from build123d import *

# Parameters (mm, degrees)
SKETCH1_W           = 150
SKETCH1_H           = 220
SKETCH1_R           = 2
SKETCH1_R_2         = 4
SKETCH1_W_2         = 25
SKETCH1_H_2         = 120
BOSS_EXTRUDE1_DEPTH = 12
SKETCH2_R           = 2
CUT_EXTRUDE1_DEPTH  = 12


with BuildPart() as part:
    # Sketch1 → Boss-Extrude1 (new body)
    with BuildSketch(Plane(origin=(0, 0, 0), x_dir=(1, 0, 0), z_dir=(0, 1, 0))):
        Rectangle(SKETCH1_W, SKETCH1_H)
        with Locations(Location((-40, 34.75, 0), (0, 0, 270))):
            Circle(SKETCH1_R, mode=Mode.SUBTRACT)
        with Locations(Location((-40, -34.75, 0), (0, 0, 270))):
            Circle(SKETCH1_R, mode=Mode.SUBTRACT)
        with Locations(Location((-50, 90, 0), (0, 0, 270))):
            Circle(SKETCH1_R_2, mode=Mode.SUBTRACT)
        with Locations(Location((50, 90, 0), (0, 0, 270))):
            Circle(SKETCH1_R_2, mode=Mode.SUBTRACT)
        with Locations(Location((-50, -90, 0), (0, 0, 270))):
            Circle(SKETCH1_R_2, mode=Mode.SUBTRACT)
        with Locations(Location((50, -90, 0), (0, 0, 270))):
            Circle(SKETCH1_R_2, mode=Mode.SUBTRACT)
        with Locations((8, 0)):
            Rectangle(SKETCH1_W_2, SKETCH1_H_2, mode=Mode.SUBTRACT)
    extrude(amount=BOSS_EXTRUDE1_DEPTH)

    # Sketch2 → Cut-Extrude1 (cut)
    with BuildSketch(Plane(origin=(0, 12, 0), x_dir=(1, 0, 0), z_dir=(0, 1, 0))):
        with Locations(Location((32.75, 26.5, 0), (0, 0, 270))):
            Circle(SKETCH2_R)
        with Locations(Location((32.75, -5.5, 0), (0, 0, 270))):
            Circle(SKETCH2_R)
    extrude(amount=-CUT_EXTRUDE1_DEPTH, mode=Mode.SUBTRACT)


solid = part.part
For this review, take the finished solid that the model builds, in its own axes (mm). A direction names the side the tool comes from. Give positions to 0.01 mm unless a question says otherwise; leave off trailing zeros. Order: outer loops, then holes, each group sorted by start corner. A loop starts at its lowest first (then second) coordinate and runs counter-clockwise, first axis right, second up. Notation, with made-up numbers: M 45,46 L 68,46 A26 ccw 68,74 Z; hole C -33,60 d11. An arc over 180 degrees is marked long. Answer in a Markdown table with one row per item. Add a question column.
(1) Mouldability with a two-part tool opening along Z and no side actions: class faces 1 (the face through (-1, 6, -110)), 2 (the face through (75, 6, 2)), 3 (the face through (20.5, 6, 1)) as +Z half, -Z half, draft (parallel to the pull), parting line (faces both ways), or undercut.
(2) For faces 4 (the face through (8, 6, -60)), 5 (the face through (-18, 12, -2)), list the 3-axis set-ups (+Z, -Z, +X, -X, +Y, -Y) from which the entire face can be reached by the end or side of a thin tool; tool diameter is ignored.
(3) Consider section A-A on z = -90. State the section outline as (x, y) points, and give its area (3 significant figures).
(4) Consider section C-C on z = 47. State the section outline as (x, y) points.
(5) Consider section B-B on x = -50. State the section outline as (y, z) points.
(6) Wall thickness on probe 1 along X at (y, z) = (9.75, -26.5); probe 2 along Z at (x, y) = (1, 8.5); probe 3 along X at (y, z) = (9.75, 37): over which ranges is each line inside the solid? List them lowest first. Write a range as [from, to].
(7) Consider section D-D on x = 17.5. State the section outline as (y, z) points, and give its area (3 significant figures).
Evaluation:
| question | item | result |
|---|---|---|
| 1 | face 1 | -Z half |
| 1 | face 2 | draft |
| 1 | face 3 | undercut |
| 2 | face 4 | +Y, -Y |
| 2 | face 5 | +Z, -Z, +X, -X, +Y |
| 3 | outline | M -75,0 L -54,0 L -54,12 L -75,12 Z; M -46,0 L 46,0 L 46,12 L -46,12 Z; M 54,0 L 75,0 L 75,12 L 54,12 Z |
| 3 | area | 1,610 mm^2 |
| 4 | outline | M -75,0 L -4.5,0 L -4.5,12 L -75,12 Z; M 20.5,0 L 75,0 L 75,12 L 20.5,12 Z |
| 5 | outline | M 0,-110 L 12,-110 L 12,-94 L 0,-94 Z; M 0,-86 L 12,-86 L 12,86 L 0,86 Z; M 0,94 L 12,94 L 12,110 L 0,110 Z |
| 6 | probe 1 | x = [-75, -4.5], [20.5, 30.75], [34.75, 75] |
| 6 | probe 2 | z = [-110, -60], [60, 110] |
| 6 | probe 3 | x = [-75, -4.5], [20.5, 75] |
| 7 | outline | M 0,-110 L 12,-110 L 12,-60 L 0,-60 Z; M 0,60 L 12,60 L 12,110 L 0,110 Z |
| 7 | area | 1,200 mm^2 |
